Geometry: final body of the model. Coordinates: model frame, mm. A direction names the side the tool comes from. Coordinates: 2 decimals unless noted, no trailing zeros. Loops run counter-clockwise (first coordinate to the right, second up) from the corner with the lowest first, then second, coordinate; pieces in that order, holes last. Notation, with made-up numbers: (89, 81) - (115, 81) arc R18 ccw to (115, 113) - close; hole circle Ø10 at (89.5, -37). An arc over 180 degrees is marked (long way). Answer in a Markdown table with one row per item.
Autodesk Inventor part; units mm, degrees
ref_plane "YZ Plane" through (0, 0, 0) normal (1, 0, 0) x (0, 1, 0)
ref_plane "XZ Plane" through (0, 0, 0) normal (0, 1, 0) x (-1, 0, 0)
ref_plane "XY Plane" through (0, 0, 0) normal (0, 0, 1) x (1, 0, 0)
sketch "Sketch1" plane through (0, 0, 0) normal (0, 0, 1) x (1, 0, 0)
  line L0 (0, 0) -> (-7.9375, 0)
  line L1 (-7.9375, 0) -> (-7.9375, -1.5875)
  line L2 (-7.9375, -1.5875) -> (-3.9687, -6.153)
  line L3 (-3.9687, -6.153) -> (-3.9687, -19.05)
  line L4 (-3.9687, -19.05) -> (0, -19.05)
  line L5 (0, -19.05) -> (0, 0)
  dimension "d0" = 15.875
  dimension "d1" = 1.5875
  dimension "d2" = 19.05
  dimension "d3" = 7.9375
  dimension "d16" = 41
revolve "Revolution1" add sketch "Sketch1" angle 360 about axis through (0, -19.05, 0) along (0, 1, 0)
chamfer "Chamfer1" distance 1.016 angle 45 1 edges at (3.9688, -19.05, 0)
thread "Thread1"
sketch "Sketch2" plane through (0, 0, 0) normal (0, 1, 0) x (1, 0, 0)
  circle A0 centre (0, 0) radius 7.9375
  line L0 (-1.3748, -2.3812) -> (-2.7496, 0)
  line L1 (-2.7496, 0) -> (-1.3748, 2.3813)
  line L2 (-1.3748, 2.3813) -> (1.3748, 2.3813)
  line L3 (1.3748, 2.3813) -> (2.7496, 0)
  line L4 (2.7496, 0) -> (1.3748, -2.3813)
  line L5 (1.3748, -2.3813) -> (-1.3748, -2.3812)
  dimension "d11" = 4.7625
extrude "Extrusion1" cut sketch "Sketch2" against normal blind 3.429 contours L0 L1 L2 L3 L4 L5
sketch "Sketch3" plane through (0, -3.429, 0) normal (0, 1, 0) x (1, 0, 0)
  line L0 (-1.3748, -2.3812) -> (1.3748, -2.3813)
  line L1 (1.3748, -2.3813) -> (2.7496, 0)
  line L2 (2.7496, 0) -> (1.3748, 2.3813)
  line L3 (1.3748, 2.3813) -> (-1.3748, 2.3813)
  line L4 (-1.3748, 2.3813) -> (-2.7496, 0)
  line L5 (-2.7496, 0) -> (-1.3748, -2.3812)
  point P0 (0, 0)
extrude "Extrusion2" cut sketch "Sketch3" against normal blind 0.254 draft -83
(1) Ray query, probe 1 along Z at (x, y) = (0.75, -1.25); probe 2 along X at (y, z) = (-15.5, -2.75); probe 3 along X at (y, z) = (-10, -2.5). Return the intervals inside material, ascending.
Verdict:
| item | result |
|---|---|
| probe 1 | z = -7.9 to -2.38, 2.38 to 7.9 |
| probe 2 | x = -2.86 to 2.86 |
| probe 3 | x = -3.08 to 3.08 |
(2) First-contact query: pin 1 Ø3 at (x, y) = (-6.5, -7) entering from +Z; pin 2 Ø1.5 at (x, z) = (-1.5, -4) entering from -Y; pin 3 Ø3 at (y, z) = (-4.5, 1) entering from -X; pin 4 Ø6 at (x, y) = (-3, -13) entering from -Z. Flat tips, straight axial feed; report the tip coordinate or a pass-through.
Verdict:
| item | result |
|---|---|
| pin 1 | passes through |
| pin 2 | stops at y = -18.48 |
| pin 3 | stops at x = -6.65 |
| pin 4 | stops at z = -3.97 |
(3) Access query for faces 5 (the face through (0.86, -12.177, 3.874)), 6 (the face through (2.05, -1.69, -1.21)), 7 (the face through (2, 0, -2)). Directions: +Z, -Z, +X, -X, +Y, -Y. A direction counts if a zero-diameter tool reaches every point of the face in a straight line with its end or side. Return the directions, or none.
Verdict:
| item | result |
|---|---|
| face 5 | -Y |
| face 6 | +Y |
| face 7 | +Z, -Z, +X, -X, +Y |
(4) Pull-direction query (X, two-part tool) for faces 1 (the face through (2.072, -1.69, 1.174)), 2 (the face through (1.72, -0.8, 7.75)), 3 (the face through (-2.072, -1.69, -1.174)), 4 (the face through (0, -19.05, 0)); classes: pulls with the +X half, pulls with the -X half, needs draft (parallel to the pull), parting line crosses it, or undercut.
Verdict:
| item | result |
|---|---|
| face 1 | undercut |
| face 2 | parting line crosses it |
| face 3 | undercut |
| face 4 | needs draft |
(5) Cut plane A-A on y = -9.25. Output: boundary loops of the cut face in (x, z), then the cut area to 3 significant figures.
Verdict:
| item | result |
|---|---|
| outline | circle Ø7.94 at (0, 0) |
| area | 49.5 mm² |
